The model under review builds one solid part; all positions refer to its coordinate system, in mm. A direction names the side the tool comes from. Coordinates: 2 decimals unless noted, no trailing zeros. Order: outer loops, then holes, each group sorted by start corner. A loop starts at its lowest first (then second) coordinate and runs counter-clockwise, first axis right, second up. Notation, with made-up numbers: (-9, 51.5) -> (16, 51.5) arc R18 ccw to (16, 79.5) -> close; hole circle Ø9 at (69, 19.25). An arc over 180 degrees is marked (long way). Put each result on its own line as item: value.
from build123d import *

# Parameters (mm, degrees)
SKETCH2_R                = 150
SKETCH2_R_2              = 50
BOSS_EXTRUDE1_DEPTH      = 50
CUT_EXTRUDE1_DEPTH       = 235.520787991
FILLET1_R                = 10
CIRPATTERN1_COUNT        = 18
FILLET1_OF_CIRPATTERN1_R = 10
SKETCH6_R                = 100
CUT_EXTRUDE2_DEPTH       = 20


with BuildPart() as part:
    # Sketch2 → Boss-Extrude1 (new, symmetric)
    with BuildSketch(Plane.XY):
        Circle(SKETCH2_R)
        Circle(SKETCH2_R_2, mode=Mode.SUBTRACT)
    extrude(amount=BOSS_EXTRUDE1_DEPTH, both=True)

    # Sketch5 → Cut-Extrude1 (cut, through all)
    with BuildSketch(Plane.XY.offset(50)):
        Polygon((-20, 180), (20, 180), (10, 130), (-10, 130), align=None)
    cut_extrude1 = extrude(amount=-CUT_EXTRUDE1_DEPTH, mode=Mode.SUBTRACT)

    # Fillet1
    fillet1_edges = [part.edges().sort_by_distance(p)[0] for p in [
        (13.871446547, 149.357232736, 0),
        (-13.871446547, 149.357232736, 0),
    ]]
    fillet(fillet1_edges, radius=FILLET1_R)

    # CirPattern1: Cut-Extrude1 ×18 about axis
    cirpattern1_axis = Axis((0, 0, 0), (0, 0, 1))
    for i in range(1, CIRPATTERN1_COUNT):
        add(cut_extrude1.rotate(cirpattern1_axis, i * 360 / CIRPATTERN1_COUNT), mode=Mode.SUBTRACT)

    # Fillet1 of CirPattern1
    fillet1_of_cirpattern1_edges = [part.edges().sort_by_distance(p)[0] for p in [
        (-38.048286187, 145.0942036, 0),
        (-64.118078107, 135.605575327, 0),
        (-85.378834074, 123.330672146, 0),
        (-106.631123166, 105.497884208, 0),
        (-122.411434515, 86.691641465, 0),
        (-136.282881062, 62.665591271, 0),
        (-144.679409353, 39.596319391, 0),
        (-149.496912182, 12.274903181, 0),
        (-149.496912182, -12.274903181, 0),
        (-144.679409353, -39.596319391, 0),
        (-136.282881062, -62.665591271, 0),
        (-122.411434515, -86.691641465, 0),
        (-106.631123166, -105.497884208, 0),
        (-85.378834074, -123.330672146, 0),
        (-64.118078107, -135.605575327, 0),
        (-38.048286187, -145.0942036, 0),
        (-13.871446547, -149.357232736, 0),
        (13.871446547, -149.357232736, 0),
        (38.048286187, -145.0942036, 0),
        (64.118078107, -135.605575327, 0),
        (85.378834074, -123.330672146, 0),
        (106.631123166, -105.497884208, 0),
        (122.411434515, -86.691641465, 0),
        (136.282881062, -62.665591271, 0),
        (144.679409353, -39.596319391, 0),
        (149.496912182, -12.274903181, 0),
        (149.496912182, 12.274903181, 0),
        (144.679409353, 39.596319391, 0),
        (136.282881062, 62.665591271, 0),
        (122.411434515, 86.691641465, 0),
        (106.631123166, 105.497884208, 0),
        (85.378834074, 123.330672146, 0),
        (64.118078107, 135.605575327, 0),
        (38.048286187, 145.0942036, 0),
    ]]
    fillet(fillet1_of_cirpattern1_edges, radius=FILLET1_OF_CIRPATTERN1_R)

    # Sketch6 → Cut-Extrude2 (cut)
    with BuildSketch(Plane.XY.offset(50)):
        Circle(SKETCH6_R)
    cut_extrude2 = extrude(amount=-CUT_EXTRUDE2_DEPTH, mode=Mode.SUBTRACT)

    # Mirror1: Cut-Extrude2 across plane
    add(cut_extrude2.mirror(Plane.XY), mode=Mode.SUBTRACT)


solid = part.part
Item 1: For faces 5 (the flat face through (95.36, 96.47, 0.7)), 6 (the flat face through (-35.844, -130.672, 0.7)), 7 (the flat face through (11, -135, 1)), 8 (the flat face through (-131.1, -34.3, 0.7)), 9 (the flat face through (78.375, 110.532, 0.7)), list the 3-axis set-ups (+Z, -Z, +X, -X, +Y, -Y) from which the entire face can be reached by the end or side of a thin tool; tool diameter is ignored.
Answers below:
face 5: +Z, -Z, +Y
face 6: +Z, -Z
face 7: +Z, -Z, -Y
face 8: +Z, -Z, -X
face 9: +Z, -Z, +X
Item 2: Consider section C-C on y = -86. Write out the cut boundary in (x, z).
Answers below:
outline: (-118.61, -50) -> (-51.03, -50) -> (-51.03, -30) -> (51.03, -30) -> (51.03, -50) -> (118.61, -50) -> (118.61, 50) -> (51.03, 50) -> (51.03, 30) -> (-51.03, 30) -> (-51.03, 50) -> (-118.61, 50) -> close
Item 3: For pin 1 Ø10 at (y, z) = (68, 25) entering from +X; pin 2 Ø1 at (y, z) = (-91.5, 12.5) entering from +X; pin 3 Ø5 at (x, z) = (108, 26.5) entering from -Y; pin 4 Ø6 at (x, y) = (80, 57) entering from -Z, all flat-tipped, find the tip position at first contact; note any pin that passes through.
Answers below:
pin 1: x = 113.74
pin 2: x = 118.39
pin 3: y = -101.88
pin 4: z = -50
Item 4: Consider section B-B on y = -40.5. Write out the cut boundary in (x, z), and give its area (3 significant figures).
Answers below:
outline: (-141.03, -50) -> (-91.43, -50) -> (-91.43, -30) -> (-29.32, -30) -> (-29.32, 30) -> (-91.43, 30) -> (-91.43, 50) -> (-141.03, 50) -> close; (29.32, -30) -> (91.43, -30) -> (91.43, -50) -> (141.03, -50) -> (141.03, 50) -> (91.43, 50) -> (91.43, 30) -> (29.32, 30) -> close
area: 17,400 mm^2
Item 5: Mouldability with a two-part tool opening along Y and no side actions: class faces 1 (the cylindrical face through (81.825, -122.489, 0.7)), 2 (the cylindrical face through (95.38, 30.04, 40.14)), 3 (the cylindrical face through (65.37, -132.16, 0.7)), 4 (the cylindrical face through (-106.632, 101.833, 0.7)) as +Y half, -Y half, draft (parallel to the pull), parting line (faces both ways), or undercut.
Answers below:
face 1: undercut
face 2: undercut
face 3: -Y half
face 4: +Y half
Item 6: Consider section A-A on x = 0. Write out the cut boundary in (y, z).
Answers below:
outline: (-130, -50) -> (-100, -50) -> (-100, -30) -> (-50, -30) -> (-50, 30) -> (-100, 30) -> (-100, 50) -> (-130, 50) -> close; (50, -30) -> (100, -30) -> (100, -50) -> (130, -50) -> (130, 50) -> (100, 50) -> (100, 30) -> (50, 30) -> close
Item 7: For line 1 (X direction, y = 129, z = -29.5); line 2 (X direction, y = 0, z = 10); line 3 (Y direction, x = 0, z = -42.5), list the stretches that pass through material, from the lowest coordinate up. Write a range as from..to.
Answers below:
line 1: -76.54..-60.26, -35.59..35.59, 60.26..76.54
line 2: -150..-50, 50..150
line 3: -130..-100, 100..130
